Verification items for this drawing (mm, ordinates from the low corner). A direction names the side the tool comes from. Round coordinates to 2 decimals unless told otherwise and drop trailing zeros. Loops run counter-clockwise (first coordinate to the right, second up) from the corner with the lowest first, then second, coordinate; pieces in that order, holes last. Notation, with made-up numbers: M -33.75,31 L 18.25,31 A23 cw 18.25,44 Z; hole C -21.75,33.5 d8. An arc over 180 degrees is marked long. One line per item, written item: value.
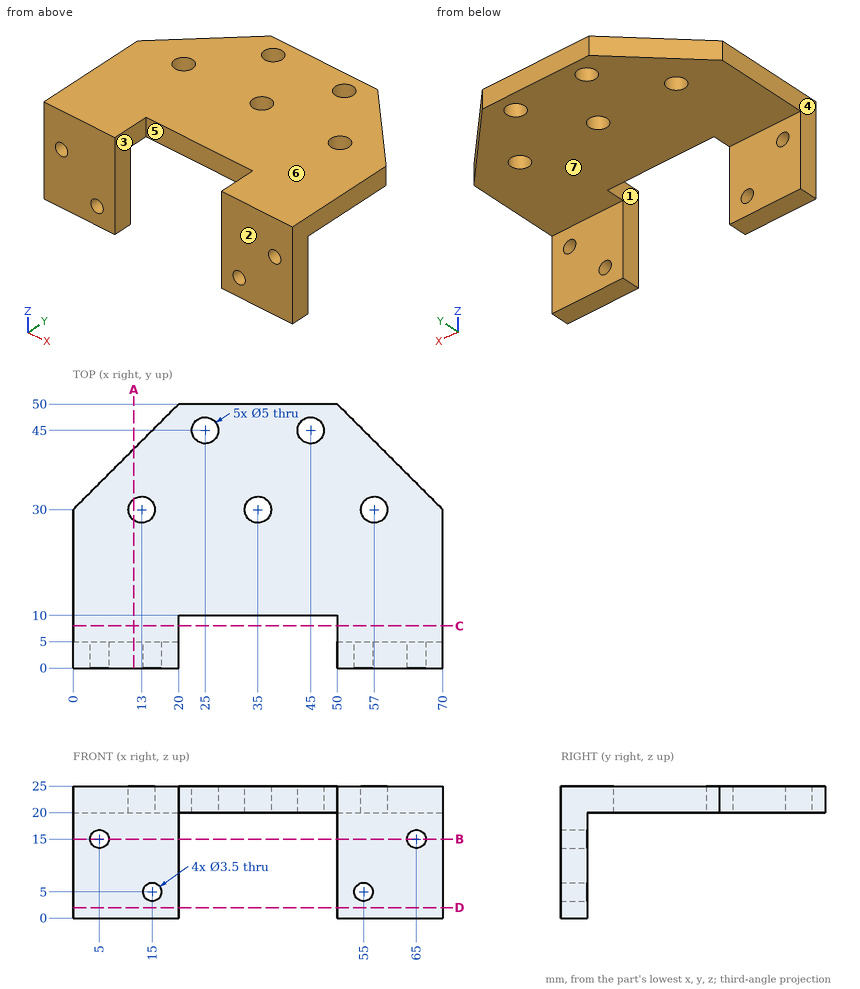
(1) Sectioned sample at A-A on x = 11.5. Enter the section's corners in (y, z), and give its area (4 significant figures).
Completed:
outline: M 0,0 L 5,0 L 5,20 L 28,20 L 28,25 L 0,25 Z; M 32,20 L 41.5,20 L 41.5,25 L 32,25 Z
area: 287.5 mm^2
(2) Tool access check on the marked faces 5, 6 and 7. Record the directions out of +Z, -Z, +X, -X, +Y, -Y that give a thin tool (end or side, any length) a straight path to the whole face; none if there is none.
Completed:
face 5: +Z, -Z, -Y
face 6: +Z, +X, -X, +Y, -Y
face 7: -Z, +X, -X, +Y
(3) Sectioned sample at D-D on z = 2. Enter the section's corners in (x, y), and give its area (3 significant figures).
Completed:
outline: M 0,0 L 20,0 L 20,5 L 0,5 Z; M 50,0 L 70,0 L 70,5 L 50,5 Z
area: 200 mm^2
(4) Sectioned sample at C-C on y = 8. Enter the section's corners in (x, z), and give its area (3 significant figures).
Completed:
outline: M 0,20 L 20,20 L 20,25 L 0,25 Z; M 50,20 L 70,20 L 70,25 L 50,25 Z
area: 200 mm^2
(5) Sectioned sample at B-B on z = 15. Enter the section's corners in (x, y).
Completed:
outline: M 0,0 L 3.25,0 L 3.25,5 L 0,5 Z; M 6.75,0 L 20,0 L 20,5 L 6.75,5 Z; M 50,0 L 63.25,0 L 63.25,5 L 50,5 Z; M 66.75,0 L 70,0 L 70,5 L 66.75,5 Z
(6) Thickness scan on L1, parallel to X at y = 3.6, z = 5; L2, parallel to X at y = 1.75, z = 15; L3, parallel to Z at x = 65, y = 3. Record the ranges inside material, lowest first. Write a range as from..to.
Completed:
L1: x = 0..13.25, 16.75..20, 50..53.25, 56.75..70
L2: x = 0..3.25, 6.75..20, 50..63.25, 66.75..70
L3: z = 0..13.25, 16.75..25
(7) Mould release check, pull along X, two halves, no side actions. Record for the marked faces 1, 2, 3 and 4: +X half, -X half, draft (parallel to the pull), parting line (faces both ways), or undercut.
Completed:
face 1: undercut
face 2: draft
face 3: undercut
face 4: -X half
(8) Depth check by flat-ended pin: pin 1 Ø3 at (x, z) = (15, 5) entering from -Y; pin 2 Ø5.5 at (x, z) = (55, 5) entering from +Y; pin 3 Ø13.5 at (x, y) = (31, 29.5) entering from -Z; pin 4 Ø5.5 at (x, z) = (28, 23.5) entering from -Y. Enter the tip coordinate at first touch or a pass-through.
Completed:
pin 1: passes through
pin 2: stops at y = 5
pin 3: stops at z = 20
pin 4: stops at y = 10
